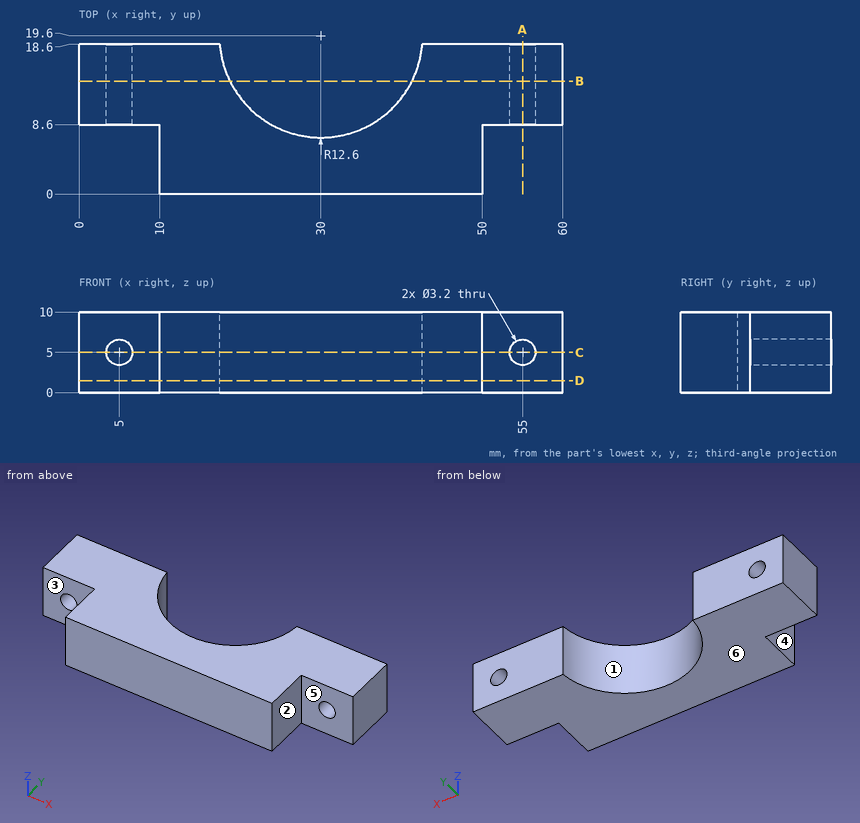
For this review, use the dimensioned drawing (mm, ordinates from the lowest corner) and the shaded views. A direction names the side the tool comes from. Give positions to 0.01 mm unless a question says otherwise; leave off trailing zeros. Order: outer loops, then holes, each group sorted by start corner. A loop starts at its lowest first (then second) coordinate and runs counter-clockwise, first axis right, second up.
1. For pin 1 Ø3 at (x, z) = (36.5, 3) entering from +Y; pin 2 Ø4.5 at (y, z) = (5, 6.5) entering from -X; pin 3 Ø3 at (x, z) = (55, 5) entering from -Y; pin 4 Ø4.5 at (y, z) = (5, 5.5) entering from +X, all flat-tipped, find the tip position at first contact; note any pin that passes through.
Solution:
pin 1: stops at y = 9.87
pin 2: stops at x = 10
pin 3: passes through
pin 4: stops at x = 50
2. Add section D-D, the plane z = 1.5. State the section outline as (x, y) points, then the cut area to 3 significant figures.
Solution:
outline: (0, 8.6) - (10, 8.6) - (10, 0) - (50, 0) - (50, 8.6) - (60, 8.6) - (60, 18.6) - (42.56, 18.6) arc R12.6 cw to (17.44, 18.6) - (0, 18.6) - close
area: 720 mm2
3. To check wall thickness, follow L1, parallel to X at y = 14, z = 5; L2, parallel to Z at x = 5, y = 10.5; L3, parallel to X at y = 12, z = 5.75. State the ranges of each line that lie inside material, in increasing order.
Solution:
L1: x = 0 to 3.4, 6.6 to 18.71, 41.29 to 53.4, 56.6 to 60
L2: z = 0 to 3.4, 6.6 to 10
L3: x = 0 to 3.59, 6.41 to 19.95, 40.05 to 53.59, 56.41 to 60
4. Add section A-A, the plane x = 55. State the section outline as (y, z) points.
Solution:
outline: (8.6, 0) - (18.6, 0) - (18.6, 3.4) - (8.6, 3.4) - close; (8.6, 6.6) - (18.6, 6.6) - (18.6, 10) - (8.6, 10) - close
5. Tool access review of the marked faces 5 and 6: name each direction out of +Z, -Z, +X, -X, +Y, -Y from which nothing blocks a thin tool from reaching the whole face with its end or side.
Solution:
face 5: +Z, -Z, +X, -Y
face 6: -Z, +X, -X, +Y, -Y
6. Mouldability with a two-part tool opening along X and no side actions: class the marked faces 1, 2, 3 and 4 as +X half, -X half, draft (parallel to the pull), parting line (faces both ways), or undercut.
Solution:
face 1: undercut
face 2: +X half
face 3: draft
face 4: -X half
7. Add section C-C, the plane z = 5. State the section outline as (x, y) points.
Solution:
outline: (0, 8.6) - (3.4, 8.6) - (3.4, 18.6) - (0, 18.6) - close; (6.6, 8.6) - (10, 8.6) - (10, 0) - (50, 0) - (50, 8.6) - (53.4, 8.6) - (53.4, 18.6) - (42.56, 18.6) arc R12.6 cw to (17.44, 18.6) - (6.6, 18.6) - close; (56.6, 8.6) - (60, 8.6) - (60, 18.6) - (56.6, 18.6) - close
8. Add section B-B, the plane y = 14. State the section outline as (x, z) points.
Solution:
outline: (0, 0) - (18.71, 0) - (18.71, 10) - (0, 10) - close; (41.29, 0) - (60, 0) - (60, 10) - (41.29, 10) - close; hole circle Ø3.2 at (5, 5); hole circle Ø3.2 at (55, 5)
